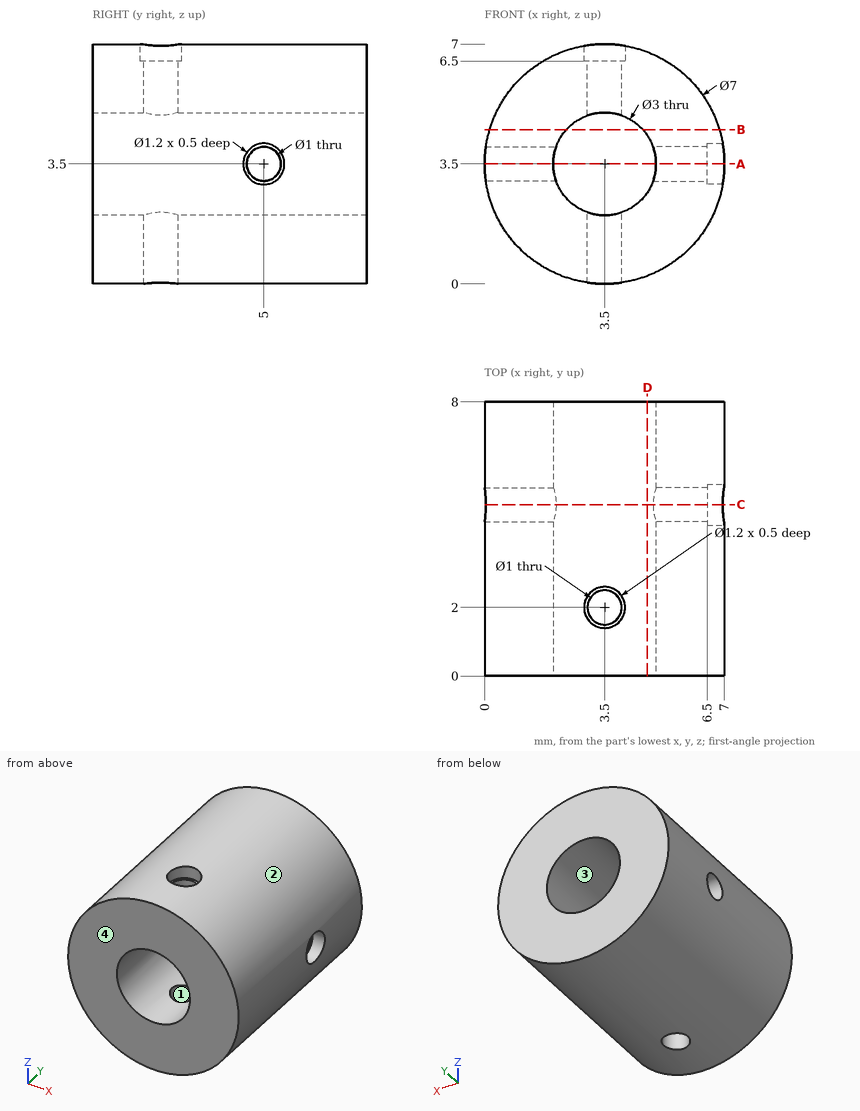
The drawing under review shows one solid part. Ordinate dimensions are in mm from its lowest x, y, z. Round coordinates to 2 decimals unless told otherwise and drop trailing zeros. Loops run counter-clockwise (first coordinate to the right, second up) from the corner with the lowest first, then second, coordinate; pieces in that order, holes last. Notation, with made-up numbers: (-1, 84) - (40, 84) arc R32 ccw to (40, 110) - close; hole circle Ø10 at (-6, -36). An arc over 180 degrees is marked (long way). One line per item, written item: value. Start each with the question number.
1) Consider section A-A on z = 3.5. Give the boundary of the cut face in (x, y).
2) Consider section B-B on z = 4.5. Give the boundary of the cut face in (x, y).
3) Draft analysis for pull direction X (two halves, no side actions). For the marked faces 1, 2, 3 and 4, state which applies: +X half, -X half, draft (parallel to the pull), parting line (faces both ways), or undercut.
4) Insertion check: pin 1 Ø4 at (y, z) = (1, 1) entering from -X; pin 2 Ø1 at (y, z) = (7, 5.5) entering from -X. Each pin has a flat end and moves straight along its axis. Give the tip position at first contact, or say it passes through.
5) Consider section D-D on x = 4.75. Give the boundary of the cut face in (y, z), then the cut area to 3 significant figures.
6) To check wall thickness, follow L1, parallel to Y at x = 6.65, z = 3.5; L2, parallel to X at y = 3.5, z = 3.5; L3, parallel to Y at x = 6.25, z = 3.5. State the ranges of each line that lie inside material, in increasing order. Write a range as from..to.
7) Consider section C-C on y = 5. Give the boundary of the cut face in (x, z).
Reported:
1. outline: (0, 0) - (2, 0) - (2, 4.5) - (0, 4.5) - close; (0, 5.5) - (2, 5.5) - (2, 8) - (0, 8) - close; (5, 0) - (7, 0) - (7, 4.4) - (6.5, 4.4) - (6.5, 4.5) - (5, 4.5) - close; (5, 5.5) - (6.5, 5.5) - (6.5, 5.6) - (7, 5.6) - (7, 8) - (5, 8) - close
2. outline: (0.15, 0) - (2.38, 0) - (2.38, 8) - (0.15, 8) - close; (4.62, 0) - (6.85, 0) - (6.85, 8) - (4.62, 8) - close
3. face 1: undercut
3. face 2: parting line
3. face 3: undercut
3. face 4: draft
4. pin 1: stops at x = 0.04
4. pin 2: stops at x = 0.34
5. outline: (0, 0.23) - (8, 0.23) - (8, 2.67) - (0, 2.67) - close; (0, 4.33) - (8, 4.33) - (8, 6.77) - (0, 6.77) - close
5. area: 39.0 mm^2
6. L1: y = 0..4.4, 5.6..8
6. L2: x = 0..2, 5..7
6. L3: y = 0..4.5, 5.5..8
7. outline: (0.04, 3) arc R3.5 ccw to (6.95, 2.9) - (6.5, 2.9) - (6.5, 3) - (4.91, 3) arc R1.5 cw to (2.09, 3) - close; (0.04, 4) - (2.09, 4) arc R1.5 cw to (4.91, 4) - (6.5, 4) - (6.5, 4.1) - (6.95, 4.1) arc R3.5 ccw to start
